Build history of the part. All positions in model axes, mm. Face numbers are marked on the shaded views. A direction names the side the tool comes from. Give positions to 0.01 mm unless a question says otherwise; leave off trailing zeros. Write each loop counter-clockwise with the first axis right and the second up, starting at its lowest first coordinate (ties: lowest second). Pieces come first, ordered by that corner, then holes.
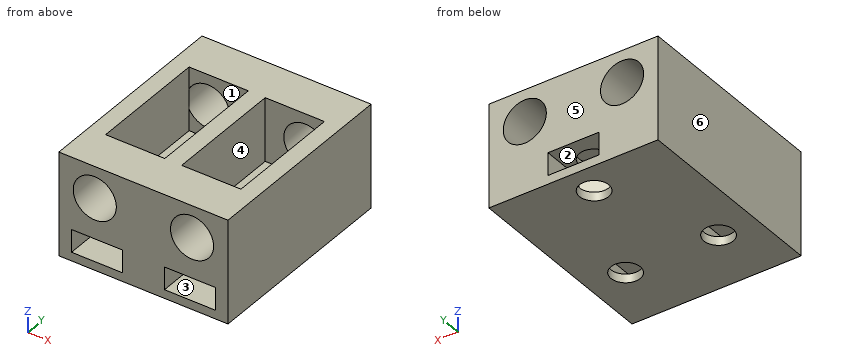
from build123d import *

# Parameters (mm, degrees)
F0_W           = 25.4
F0_H           = 9.525
F1_DEPTH       = 6.35
F2_W           = 2.54
F2_H           = 9.525
F3_DEPTH       = 17.78
F4_W           = 25.4
F4_H           = 9.525
F5_DEPTH       = 6.35
F6_R           = 3.2385
F7_DEPTH       = 6.35
F8_R           = 3.2385
F9_DEPTH       = 6.35
F10_W          = 25.4
F10_H          = 30.48
F11_DEPTH      = 6
F14_DEPTH      = 1.7
F14_DEPTH_BACK = 1.7
F15_R          = 2.2
F16_DEPTH      = 5.588


with BuildPart() as f1:
    # F0 (on Front) → F1 (new body)
    with BuildSketch(Plane.XZ):
        Rectangle(F0_W, F0_H)
    extrude(amount=F1_DEPTH)

    # F2 (on face) → F3 (join)
    with BuildSketch(Plane.XZ.offset(6.35)):
        with Locations((-11.43, 0)):
            Rectangle(F2_W, F2_H)
        Rectangle(F2_W, F2_H)
        with Locations((11.43, 0)):
            Rectangle(F2_W, F2_H)
    extrude(amount=F3_DEPTH)

    # F4 (on face) → F5 (join)
    with BuildSketch(Plane.XZ.offset(24.13)):
        Rectangle(F4_W, F4_H)
    extrude(amount=F5_DEPTH)

    # F6 (on face) → F7 (cut, through all)
    with BuildSketch(Plane(origin=(0, 0, 0), x_dir=(-1, 0, 0), z_dir=(0, 1, 0))):
        with Locations((7.3025, 0)):
            Circle(F6_R)
        with Locations((-7.3025, 0)):
            Circle(F6_R)
    extrude(amount=-F7_DEPTH, mode=Mode.SUBTRACT)

    # F8 (on face) → F9 (cut, through all)
    with BuildSketch(Plane.XZ.offset(30.48)):
        with Locations((-7.3025, 0)):
            Circle(F8_R)
        with Locations((7.3025, 0)):
            Circle(F8_R)
    extrude(amount=-F9_DEPTH, mode=Mode.SUBTRACT)

    # F10 (on face) → F11 (join)
    with BuildSketch(Plane(origin=(0, 0, -4.7625), x_dir=(1, 0, 0), z_dir=(0, 0, -1))):
        with Locations((0, 15.24)):
            Rectangle(F10_W, F10_H)
    extrude(amount=F11_DEPTH)

    # F13 (on offset) → F14 (cut, two sides)
    with BuildSketch(Plane(origin=(0, 0, -7.7625), x_dir=(1, 0, 0), z_dir=(0, 0, -1))) as f14_sk:
        Polygon((-3.16, 18.8017653474), (-3.16, 23.2098346526), (-3.16, 30.48), (-10.795, 30.48), (-10.795, 23.2098346526), (-10.795, 18.8017653474), (-6.9775, 16.5977306947), align=None)
        Polygon((10.795, 18.8017653474), (10.795, 23.2098346526), (10.795, 30.48), (3.16, 30.48), (3.16, 23.2098346526), (3.16, 18.8017653474), (6.9775, 16.5977306947), align=None)
        Polygon((3.8175, 2.2040346526), (3.8175, 6.6121039579), (0, 8.8161386105), (-3.8175, 6.6121039579), (-3.8175, 2.2040346526), (-3.8175, -0.0115306947), (3.8175, -0.0115306947), align=None)
    extrude(amount=-F14_DEPTH, mode=Mode.SUBTRACT)
    extrude(f14_sk.sketch, amount=F14_DEPTH_BACK, mode=Mode.SUBTRACT)

    # F15 (on face) → F16 (cut)
    with BuildSketch(Plane(origin=(0, 0, -10.7625), x_dir=(1, 0, 0), z_dir=(0, 0, -1))):
        with Locations((0, 4.4080693053)):
            Circle(F15_R)
        with Locations((6.9775, 21.0058)):
            Circle(F15_R)
        with Locations((-6.9775, 21.0058)):
            Circle(F15_R)
    extrude(amount=-F16_DEPTH, mode=Mode.SUBTRACT)


solid = f1.part
(1) Probe line 1 (X direction, y = -11.5, z = -0.5); line 2 (X direction, y = -26, z = 0); line 3 (Z direction, x = -9.5, y = -19.5). List the from-to ranges inside material, lowest first.
(2) 3-axis set-ups, long thin cutter, end or side, ignore diameter. For the marked faces 1, 2 and 3: which of +Z, -Z, +X, -X, +Y, -Y reach the whole face in a straight line?
(3) Saw through at B-B, the plane y = -15.5. List the corners of the cut face in (x, z), plus the area to 3 significant figures.
(4) Saw through at A-A, the plane z = 0. List the corners of the cut face in (x, y).
(5) Saw through at C-C, the plane x = 6. List the corners of the cut face in (y, z), plus the area to 3 significant figures.
(6) Drop flat-ended pins along their axis: pin 1 (1.3 mm diameter, centred on x = -1, y = -3.5, fed in from -Z); pin 2 (2.5 mm diameter, centred on x = 6.98, y = -21.01, fed in from +Z). Give the stop position or say it passes through.
(7) Saw through at D-D, the plane z = -9. List the corners of the cut face in (x, y) (1 decimal), plus the area to 3 significant figures.
(8) Mould opens along Y. For the marked faces 4, 5 and 6 say: +Y half, -Y half, draft (parallel to the pull), parting line (faces both ways), or undercut.
Computed values:
1. line 1: x = -12.7 to -10.16, -1.27 to 1.27, 10.16 to 12.7
1. line 2: x = -12.7 to -10.54, -4.06 to 4.06, 10.54 to 12.7
1. line 3: z = -10.76 to -9.46, -6.06 to -4.76
2. face 1: +Z
2. face 2: +Y
2. face 3: -Y
3. outline: (-12.7, -10.76) - (12.7, -10.76) - (12.7, 4.76) - (10.16, 4.76) - (10.16, -4.76) - (1.27, -4.76) - (1.27, 4.76) - (-1.27, 4.76) - (-1.27, -4.76) - (-10.16, -4.76) - (-10.16, 4.76) - (-12.7, 4.76) - close
3. area: 225 mm2
4. outline: (-12.7, -30.48) - (-10.54, -30.48) - (-10.54, -24.13) - (-10.16, -24.13) - (-10.16, -6.35) - (-10.54, -6.35) - (-10.54, 0) - (-12.7, 0) - close; (-4.06, -30.48) - (4.06, -30.48) - (4.06, -24.13) - (1.27, -24.13) - (1.27, -6.35) - (4.06, -6.35) - (4.06, 0) - (-4.06, 0) - (-4.06, -6.35) - (-1.27, -6.35) - (-1.27, -24.13) - (-4.06, -24.13) - close; (10.16, -24.13) - (10.54, -24.13) - (10.54, -30.48) - (12.7, -30.48) - (12.7, 0) - (10.54, 0) - (10.54, -6.35) - (10.16, -6.35) - close
5. outline: (-30.48, -10.76) - (-22.98, -10.76) - (-22.98, -9.46) - (-30.48, -9.46) - close; (-30.48, -6.06) - (-22.98, -6.06) - (-22.98, -5.17) - (-19.03, -5.17) - (-19.03, -6.06) - (-17.16, -6.06) - (-17.16, -9.46) - (-19.03, -9.46) - (-19.03, -10.76) - (0, -10.76) - (0, -2.97) - (-6.35, -2.97) - (-6.35, -4.76) - (-24.13, -4.76) - (-24.13, -2.97) - (-30.48, -2.97) - close; (-30.48, 2.97) - (-24.13, 2.97) - (-24.13, 4.76) - (-30.48, 4.76) - close; (-6.35, 2.97) - (0, 2.97) - (0, 4.76) - (-6.35, 4.76) - close
5. area: 175 mm2
6. pin 1: stops at z = -5.17
6. pin 2: stops at z = -4.76
7. outline: (-12.7, -30.5) - (-10.8, -30.5) - (-10.8, -18.8) - (-7, -16.6) - (-3.2, -18.8) - (-3.2, -30.5) - (3.2, -30.5) - (3.2, -18.8) - (7, -16.6) - (10.8, -18.8) - (10.8, -30.5) - (12.7, -30.5) - (12.7, 0) - (3.8, 0) - (3.8, -6.6) - (0, -8.8) - (-3.8, -6.6) - (-3.8, 0) - (-12.7, 0) - close
7. area: 520 mm2
8. face 4: undercut
8. face 5: +Y half
8. face 6: draft
